Check sheet for the modelled part. Datum: model origin and axes. Units: mm. A direction names the side the tool comes from. Round coordinates to 2 decimals unless told otherwise and drop trailing zeros. Write each loop counter-clockwise with the first axis right and the second up, starting at its lowest first coordinate (ties: lowest second). Pieces come first, ordered by that corner, then holes. Notation, with made-up numbers: (1.5, 75) -> (5.5, 75) arc R32 cw to (5.5, 105) -> close; hole circle Ø7 at (68.25, 29.5). An arc over 180 degrees is marked (long way). One line per item, written item: value.
Autodesk Inventor part; units mm, degrees
ref_plane "Work Plane1" through (20, 42.75, -18) normal (0, 1, 0) x (-1, 0, 0)
ref_plane "YZ Plane" through (0, 0, 0) normal (1, 0, 0) x (0, 1, 0)
ref_plane "XZ Plane" through (0, 0, 0) normal (0, 1, 0) x (-1, 0, 0)
sketch "Sketch1" plane through (0, 0, 0) normal (1, 0, 0) x (0, 1, 0)
  line L0 (0, 0) -> (35, 0)
  line L1 (35, 0) -> (35, 27)
  line L2 (35, 27) -> (0, 27)
  line L3 (0, 27) -> (0, 0)
  line L4 (0, 27) -> (25, 27) construction
  line L5 (25, 27) -> (25, 0) construction
  line L6 (25, 0) -> (0, 0) construction
  line L7 (0, 0) -> (0, 27) construction
  circle A0 centre (12.5, 12.5) radius 6.35
  dimension "d0" = 35
  dimension "d1" = 27
  dimension "d2" = 25
  dimension "d3" = 12.7
extrude "Extrusion1" add sketch "Sketch1" along normal blind 10
sketch "Sketch2" plane through (10, 0, 0) normal (1, 0, 0) x (0, 0, -1)
  line L0 (0, 35) -> (-27, 35)
  line L1 (0, 0) -> (0, 35)
  line L2 (-27, 35) -> (0, 35)
  line L3 (0, 35) -> (0, 25)
  line L4 (0, 25) -> (-27, 25)
  line L5 (-27, 25) -> (-27, 35)
  dimension "d6" = 10
extrude "Extrusion2" add sketch "Sketch2" along normal blind 10
sketch "Sketch3" plane through (10, 0, 0) normal (1, 0, 0) x (0, 0, -1)
  point P0 (0, 0)
sketch "Sketch4" plane through (0, 0, 0) normal (0, 0, -1) x (-1, 0, 0)
  point P0 (0, 0)
sketch "Sketch5" plane through (10, 0, 0) normal (1, 0, 0) x (0, 0, -1)
  point P0 (0, 0)
sketch "Sketch6" plane through (10, 0, 0) normal (1, 0, 0) x (0, 0, -1)
  line L0 (-27, 25) -> (-27, 0)
  line L1 (-27, 0) -> (-22, 0)
  line L2 (-22, 0) -> (-22, 11)
  line L3 (-22, 11) -> (-27, 11)
  line L4 (-27, 11) -> (-27, 0)
  line L5 (-22, 14) -> (-27, 14)
  line L6 (-27, 14) -> (-27, 19)
  line L7 (-27, 19) -> (-22, 19)
  line L8 (-22, 19) -> (-22, 14)
  point P0 (0, 0)
  dimension "d9" = 5
  dimension "d10" = 11
  dimension "d11" = 5
extrude "Extrusion3" add sketch "Sketch6" along normal blind 150
sketch "Sketch7" plane through (10, 19, 27) normal (0, 1, 0) x (1, 0, 0)
  line L0 (-10, 0) -> (10, 0)
  line L1 (0, 5) -> (150, 5)
  line L2 (0, 0) -> (10, 0)
  line L3 (10, 0) -> (10, 5)
  line L4 (10, 5) -> (0, 5)
  line L5 (0, 5) -> (0, 0)
  point P0 (-10, 27)
  dimension "d14" = 10
extrude "Extrusion4" add sketch "Sketch7" along normal blind 7.5
sketch "Sketch8" plane through (160, 0, 0) normal (1, 0, 0) x (0, 0, -1)
  line L0 (-27, 14) -> (-22, 14)
  line L1 (-27, 14) -> (-22, 14)
  line L2 (-22, 25) -> (-22, 14)
  line L3 (-22, 14) -> (-22, 25)
  line L4 (-22, 25) -> (0, 25)
  line L5 (-22, 25) -> (0, 25)
  line L6 (0, 25) -> (0, 35)
  line L7 (0, 25) -> (0, 35)
  line L8 (0, 35) -> (-27, 35)
  line L9 (-27, 35) -> (-27, 14)
  line L10 (-22, 11) -> (-22, 0)
  line L11 (-27, 0) -> (-22, 0)
  line L12 (-22, 0) -> (-22, 11)
  line L13 (-22, 11) -> (-27, 11)
  line L14 (-27, 11) -> (-27, 0)
  point P0 (0, 0)
extrude "Extrusion5" add sketch "Sketch8" along normal blind 10
sketch "Sketch9" plane through (170, 0, 0) normal (1, 0, 0) x (0, 0, -1)
  line L0 (0, 35) -> (-27, 35)
  line L1 (-27, 35) -> (0, 35)
  line L2 (0, 35) -> (0, 0)
  line L3 (0, 0) -> (-27, 0)
  line L4 (-27, 0) -> (-27, 35)
  circle A0 centre (-12.5, 12.5) radius 6.35
  circle A1 centre (-12.5, 12.5) radius 6.35
extrude "Extrusion6" add sketch "Sketch9" along normal blind 10
fillet "Fillet1" radius 2 2 edges at (90, 11, 22) (90, 14, 22)
sketch "Sketch10" plane through (20, 0, 0) normal (1, 0, 0) x (0, 0, -1)
  line L0 (0, 35) -> (-27, 35)
  line L1 (-13.5, 35) -> (-20.5, 35)
  line L2 (-20.5, 35) -> (-6.5, 35)
  line L3 (-20.5, 35) -> (-6.5, 35)
  line L4 (-6.5, 35) -> (-6.5, 32)
  line L5 (-6.5, 32) -> (-20.5, 32)
  line L6 (-20.5, 32) -> (-20.5, 35)
  point P0 (0, 0)
  dimension "d22" = 7
  dimension "d23" = 14
  dimension "d24" = 3
extrude "Extrusion7" add sketch "Sketch10" along normal blind 140
sketch "Sketch11" plane through (0, 35, 27) normal (0, 1, 0) x (1, 0, 0)
  point P0 (0, 27)
sketch "Sketch12" plane through (160, 25, 0) normal (0, 0, -1) x (-1, 0, 0)
  line L0 (-4, 3.5) -> (-16, 3.5)
  line L1 (-16, 3.5) -> (-16, 6.5)
  line L2 (-16, 6.5) -> (-4, 6.5)
  line L3 (-4, 6.5) -> (-4, 3.5)
  line L4 (-4, 3.5) -> (-16, 6.5) construction
  line L5 (-16, 3.5) -> (-4, 6.5) construction
  line L6 (156, 6.5) -> (144, 6.5)
  line L7 (144, 6.5) -> (144, 3.5)
  line L8 (144, 3.5) -> (156, 3.5)
  line L9 (156, 3.5) -> (156, 6.5)
  line L10 (156, 6.5) -> (144, 3.5) construction
  line L11 (144, 6.5) -> (156, 3.5) construction
  point P0 (160, -25)
  point P1 (-10, 5)
  point P2 (150, 5)
  dimension "d27" = 12
  dimension "d28" = 3
  dimension "d29" = 12
  dimension "d30" = 3
extrude "Extrusion8" cut sketch "Sketch12" against normal blind 23.5
sketch "Sketch13" plane through (0, 0, 0) normal (-1, 0, 0) x (0, 0, 1)
  circle A0 centre (12.5, 12.5) radius 6.35 construction
  circle A1 centre (12.5, 12.5) radius 20.6375 construction
  point P0 (0, 0)
  dimension "d33" = 41.275
sketch "Sketch14" plane through (170, 0, 0) normal (-1, 0, 0) x (0, 0, 1)
  circle A0 centre (12.5, 12.5) radius 6.35
  circle A1 centre (12.5, 12.5) radius 6.35
  circle A2 centre (12.5, 12.5) radius 3.5
  point P0 (0, 0)
  dimension "d34" = 7
extrude "Extrusion9" add sketch "Sketch14" against normal blind 4.5
sketch "Sketch15" plane through (10, 0, 0) normal (1, 0, 0) x (0, 0, -1)
  circle A0 centre (-12.5, 12.5) radius 3.5
  circle A1 centre (-12.5, 12.5) radius 6.35
  circle A2 centre (-12.5, 12.5) radius 3.5
  point P0 (0, 0)
  dimension "d37" = 7
extrude "Extrusion10" add sketch "Sketch15" against normal blind 4.5
sketch "Sketch16" plane through (0, 0, 27) normal (0, 0, 1) x (1, 0, 0)
  point P0 (0, 0)
sketch "Sketch17" plane through (0, 0, 27) normal (0, 0, 1) x (1, 0, 0)
  point P0 (0, 0)
sketch "Sketch18" plane through (0, 0, 27) normal (0, 0, 1) x (1, 0, 0)
  line L0 (0, 35) -> (0, 0)
  line L1 (180, 35) -> (180, 0)
  line L2 (0, 0) -> (180, 0)
  line L3 (180, 0) -> (180, 3)
  line L4 (180, 3) -> (0, 3)
  line L5 (0, 3) -> (0, 0)
  point P0 (0, 3)
  dimension "d40" = 3
extrude "Extrusion11" add sketch "Sketch18" against normal blind 67
sketch "Sketch19" plane through (0, 3, 27) normal (0, 1, 0) x (-1, 0, 0)
  line L0 (180, 0) -> (180, -42) construction
  point P0 (0, 0)
sketch "Sketch20" plane through (0, 3, -40) normal (0, 1, 0) x (1, 0, 0)
  circle A0 centre (90, -20) radius 19
  circle A1 centre (90, -20) radius 20
  circle A2 centre (50, -20) radius 20
  circle A3 centre (50, -20) radius 19
  circle A4 centre (130, -20) radius 20
  circle A5 centre (130, -20) radius 19
  point P0 (0, -40)
  point P1 (110, -20)
  point P2 (70, -20)
  dimension "d43" = 38
  dimension "d44" = 38
  dimension "d45" = 38
extrude "Extrusion12" add sketch "Sketch20" along normal blind 30
sketch "Sketch21" plane through (10, 3, 22) normal (0, 1, 0) x (1, 0, 0)
  line L0 (-10, 22) -> (-10, 62)
  line L1 (-10, 62) -> (10, 62)
  line L2 (10, 62) -> (10, 52)
  line L3 (10, 52) -> (-10, 52)
  line L4 (-10, 52) -> (-10, 62)
  line L5 (170, 62) -> (-10, 62)
  line L6 (170, 62) -> (150, 62)
  line L7 (150, 62) -> (150, 52)
  line L8 (150, 52) -> (170, 52)
  line L9 (170, 52) -> (170, 62)
  dimension "d48" = 10
  dimension "d49" = 10
extrude "Extrusion13" add sketch "Sketch21" along normal blind 32
sketch "Sketch22" plane through (4, 28.5, 0) normal (0, 1, 0) x (1, 0, 0)
  point P0 (-4, 0)
sketch "Sketch23" plane through (0, 0, -40) normal (0, 0, -1) x (-1, 0, 0)
  line L0 (-4, 28.5) -> (-16, 28.5)
  line L1 (-4, 31.5) -> (-4, 28.5)
  line L2 (-16, 28.5) -> (-4, 28.5)
  line L3 (-4, 28.5) -> (-4, 31.5)
  line L4 (-4, 31.5) -> (-16, 31.5)
  line L5 (-16, 31.5) -> (-16, 28.5)
  line L6 (-164, 28.5) -> (-176, 28.5)
  line L7 (-164, 31.5) -> (-164, 28.5)
  line L8 (-176, 28.5) -> (-164, 28.5)
  line L9 (-164, 28.5) -> (-164, 31.5)
  line L10 (-164, 31.5) -> (-176, 31.5)
  line L11 (-176, 31.5) -> (-176, 28.5)
  point P0 (0, 0)
extrude "Extrusion14" cut sketch "Sketch23" against normal blind 10
sketch "Sketch24" plane through (130, 33, -20) normal (0, 1, 0) x (1, 0, 0)
  line L0 (27.2959, -23.1323) -> (-103.8128, -23.1323)
  line L1 (-103.8128, -23.1323) -> (-103.8128, 25.7271)
  line L2 (-103.8128, 25.7271) -> (27.2959, 25.7271)
  line L3 (27.2959, 25.7271) -> (27.2959, -23.1323)
  point P0 (-130, -20)
extrude "Extrusion15" cut sketch "Sketch24" against normal blind 30
sketch "Sketch25" plane through (10, 3, 22) normal (0, 1, 0) x (1, 0, 0)
  circle A0 centre (80, 38.75) radius 19
  circle A1 centre (80, 38.75) radius 20.75
  circle A2 centre (121.5, 38.75) radius 20.75
  circle A3 centre (121.5, 38.75) radius 19
  circle A4 centre (38.5, 38.75) radius 20.75
  circle A5 centre (38.5, 38.75) radius 19
  point P0 (-10, 22)
  point P1 (59.25, 38.75)
  point P2 (100.75, 38.75)
  dimension "d56" = 38
  dimension "d57" = 41.5
  dimension "d58" = 38
  dimension "d59" = 38
extrude "Extrusion16" add sketch "Sketch25" along normal blind 45
sketch "Sketch26" plane through (0, 35, 27) normal (0, 1, 0) x (1, 0, 0)
  line L0 (20, 6.5) -> (160, 6.5)
  line L1 (20, 20.5) -> (160, 20.5)
  line L2 (20, 6.5) -> (160, 6.5)
  line L3 (160, 6.5) -> (160, 20.5)
  line L4 (160, 20.5) -> (20, 20.5)
  line L5 (20, 20.5) -> (20, 6.5)
  point P0 (0, 27)
extrude "Extrusion17" cut sketch "Sketch26" against normal blind 5
sketch "Sketch27" plane through (10, 48, 22) normal (0, 1, 0) x (1, 0, 0)
  line L0 (16.1578, 67.5748) -> (146.5005, 67.5748)
  line L1 (146.5005, 67.5748) -> (146.5005, 15.2049)
  line L2 (146.5005, 15.2049) -> (16.1578, 15.2049)
  line L3 (16.1578, 15.2049) -> (16.1578, 67.5748)
  point P0 (-10, 22)
extrude "Extrusion18" cut sketch "Sketch27" against normal blind 45
sketch "Sketch28" plane through (10, 3, 22) normal (0, 1, 0) x (1, 0, 0)
  point P0 (-10, 22)
sketch "Sketch29" plane through (0, 0, 0) normal (-1, 0, 0) x (0, 0, 1)
  point P0 (0, 0)
sketch "Sketch30" plane through (20, 3, -30) normal (1, 0, 0) x (0, 0, -1)
  circle A0 centre (-12, 19) radius 19
  line L0 (-30, 0) -> (0, 0)
  circle A1 centre (-12, 19) radius 20.75
  point P0 (-30, -3)
  point P1 (-3.6596, 0)
  point P2 (-20.3404, 0)
  point P3 (-12, 0)
  dimension "d66" = 41.5
extrude "Extrusion19" add sketch "Sketch30" along normal blind 140 contours L0 A1 picked at (-31.4706, 19.7749)
ref_plane "Work Plane1" through (20, 42.75, -18) normal (0, 1, 0) x (-1, 0, 0)
sketch "Sketch31" plane through (20, 42.75, -18) normal (0, 1, 0) x (-1, 0, 0)
  line L0 (0, -22) -> (-140, -22)
  line L1 (0, 20.75) -> (-140, 20.75)
  line L2 (-140, -22) -> (-130, -22)
  line L3 (-130, -22) -> (-130, 20.75)
  line L4 (-130, 20.75) -> (-140, 20.75)
  line L5 (-140, 20.75) -> (-140, -22)
  line L6 (-130, 20.75) -> (-120, 20.75)
  line L7 (-120, 20.75) -> (-120, -22)
  line L8 (-120, -22) -> (-130, -22)
  line L9 (-130, -22) -> (-130, 20.75)
  line L10 (-120, 20.75) -> (-110, 20.75)
  line L11 (-110, 20.75) -> (-110, -22)
  line L12 (-110, -22) -> (-120, -22)
  line L13 (-120, -22) -> (-120, 20.75)
  line L14 (-110, 20.75) -> (-100, 20.75)
  line L15 (-100, 20.75) -> (-100, -22)
  line L16 (-100, -22) -> (-110, -22)
  line L17 (-110, -22) -> (-110, 20.75)
  line L18 (-100, 20.75) -> (-90, 20.75)
  line L19 (-90, 20.75) -> (-90, -22)
  line L20 (-90, -22) -> (-100, -22)
  line L21 (-100, -22) -> (-100, 20.75)
  line L22 (-90, 20.75) -> (-80, 20.75)
  line L23 (-80, 20.75) -> (-80, -22)
  line L24 (-80, -22) -> (-90, -22)
  line L25 (-90, -22) -> (-90, 20.75)
  line L26 (-80, 20.75) -> (-70, 20.75)
  line L27 (-70, 20.75) -> (-70, -22)
  line L28 (-70, -22) -> (-80, -22)
  line L29 (-80, -22) -> (-80, 20.75)
  line L30 (-70, 20.75) -> (-60, 20.75)
  line L31 (-60, 20.75) -> (-60, -22)
  line L32 (-60, -22) -> (-70, -22)
  line L33 (-70, -22) -> (-70, 20.75)
  line L34 (-60, 20.75) -> (-50, 20.75)
  line L35 (-50, 20.75) -> (-50, -22.9756)
  line L36 (-50, -22.9756) -> (-60, -22.9756)
  line L37 (-60, -22.9756) -> (-60, 20.75)
  line L38 (-50, 20.75) -> (-40, 20.75)
  line L39 (-40, 20.75) -> (-40, -22)
  line L40 (-40, -22) -> (-50, -22)
  line L41 (-50, -22) -> (-50, 20.75)
  line L42 (-40, 20.75) -> (-30, 20.75)
  line L43 (-30, 20.75) -> (-30, -22)
  line L44 (-30, -22) -> (-40, -22)
  line L45 (-40, -22) -> (-40, 20.75)
  line L46 (-30, 20.75) -> (-20, 20.75)
  line L47 (-20, 20.75) -> (-20, -22)
  line L48 (-20, -22) -> (-30, -22)
  line L49 (-30, -22) -> (-30, 20.75)
  line L50 (-20, 20.75) -> (-10, 20.75)
  line L51 (-10, 20.75) -> (-10, -22)
  line L52 (-10, -22) -> (-20, -22)
  line L53 (-20, -22) -> (-20, 20.75)
  line L54 (-10, 20.75) -> (0, 20.75)
  line L55 (0, 20.75) -> (0, -22)
  line L56 (0, -22) -> (-10, -22)
  line L57 (-10, -22) -> (-10, 20.75)
  point P0 (20, 18)
  point P1 (-80, -22)
  point P2 (-60, -22)
  point P3 (-20, -22)
  point P4 (-10, -22)
  point P5 (-120, -22)
  point P6 (-90, -22)
  dimension "d69" = 10
  dimension "d70" = 10
  dimension "d71" = 10
  dimension "d72" = 10
  dimension "d73" = 10
  dimension "d74" = 10
  dimension "d75" = 10
  dimension "d76" = 10
  dimension "d77" = 10
  dimension "d78" = 10
  dimension "d79" = 10
  dimension "d80" = 10
  dimension "d81" = 10
extrude "Extrusion20" cut sketch "Sketch31" against normal blind 19 contours L0 L51 L1 L55 | L0 L43 L1 L47 | L0 L39 L1 L43 | L0 L35 L1 L39 | L0 L27 L1 L31 | L0 L23 L1 L27 | L0 L15 L1 L19 | L0 L11 L1 L15 | L0 L7 L1 L11 | L0 L5 L1 L3
properties part number "_3DPrint"
Item 1: Tool access check on faces 5 (the flat face through (140, 41, -15)), 6 (the flat face through (89, 19, 25)), 7 (the flat face through (160, 11, -2)), 8 (the cylindrical face through (2.712, 15.43, 18.134)), 9 (the flat face through (10, 30, 23.5)). Record the directions out of +Z, -Z, +X, -X, +Y, -Y that give a thin tool (end or side, any length) a straight path to the whole face; none if there is none.
Result set:
face 5: +Z, -Z, +Y
face 6: +Z, +Y
face 7: none
face 8: -X
face 9: -Z
Item 2: Release check for a two-part mould opening along X. For faces 1 (the flat face through (170, 28.5, 12)), 2 (the cylindrical face through (172.218, 9.083, 11.741)), 3 (the flat face through (5.5, 9.8, 9.8)), 4 (the flat face through (160, 4, -27)) record: pulls with the +X half, pulls with the -X half, needs draft (parallel to the pull), parting line crosses it, or undercut.
Result set:
face 1: undercut
face 2: needs draft
face 3: pulls with the -X half
face 4: pulls with the +X half
Item 3: Depth check by flat-ended pin: pin 1 (1.9 mm diameter, centred on x = 23, z = 2, fed in from +Y); pin 2 (9.5 mm diameter, centred on y = 37, z = -21.5, fed in from -X); pin 3 (6.5 mm diameter, centred on x = 60.5, y = 6.5, fed in from -Z); pin 4 (10 mm diameter, centred on y = 28, z = -20.5, fed in from +X) (3 decimals). Enter the tip coordinate at first touch or a pass-through.
Result set:
pin 1: y = 23.75
pin 2: x = 30
pin 3: z = -34.75
pin 4: through
Item 4: Sectioned sample at B-B (z = 12.5). State how many separate pieces and enclosed holes the cut face has, then the cut area to 3 significant figures.
Result set:
separate pieces: 3
enclosed holes: 2
area: 1,110 mm^2
Item 5: Sectioned sample at D-D (z = -15). Enter the section's corners in (x, y), then the cut area to 3 significant figures.
Result set:
outline: (0, 0) -> (180, 0) -> (180, 3) -> (160, 3) -> (160, 3.24) -> (20, 3.24) -> (20, 3) -> (0, 3) -> close; (30, 40.76) -> (40, 40.76) -> (40, 42.53) -> (30, 42.53) -> close; (70, 40.76) -> (80, 40.76) -> (80, 42.53) -> (70, 42.53) -> close; (100, 40.76) -> (110, 40.76) -> (110, 42.53) -> (100, 42.53) -> close; (140, 40.76) -> (150, 40.76) -> (150, 42.53) -> (140, 42.53) -> close
area: 644 mm^2
Item 6: Sectioned sample at C-C (x = 154). Enter the section's corners in (y, z).
Result set:
outline: (0, -40) -> (3, -40) -> (3, -26.34) arc R20.75 ccw to (23.75, -38.68) -> (23.75, -36.92) arc R19 cw (long way) to (23.75, 0.92) -> (23.75, 2.68) arc R20.75 ccw to (3, -9.66) -> (3, 22) -> (9, 22) arc R2 ccw to (11, 24) -> (11, 27) -> (0, 27) -> close; (14, 24) arc R2 ccw to (16, 22) -> (19, 22) -> (19, 27) -> (14, 27) -> close
Item 7: Sectioned sample at A-A (x = 32). Enter the section's corners in (y, z).
Result set:
outline: (0, -40) -> (3, -40) -> (3, -26.34) arc R20.75 ccw (long way) to (3, -9.66) -> (3, 22) -> (9, 22) arc R2 ccw to (11, 24) -> (11, 27) -> (0, 27) -> close; (14, 24) arc R2 ccw to (16, 22) -> (19, 22) -> (19, 27) -> (14, 27) -> close; hole circle Ø38 at (22, -18)
Item 8: Material ranges on line 1 along Z through (x, y) = (2, 12); line 2 along X through (y, z) = (32.5, -34); line 3 along Y through (x, z) = (8.3, 12.5), recorded low to high.
Result set:
line 1: -40 to -30, 0 to 6.17, 18.83 to 27
line 2: 0 to 20, 30 to 40, 70 to 80, 100 to 110, 140 to 150, 160 to 180
line 3: 0 to 9, 16 to 28.5, 31.5 to 35
